Verification items for the finished model (mm, model axes). A direction names the side the tool comes from. Give positions to 0.01 mm unless a question says otherwise; leave off trailing zeros. Loops run counter-clockwise (first coordinate to the right, second up) from the corner with the lowest first, then second, coordinate; pieces in that order, holes last. Notation, with made-up numbers: M 40,63 L 96,63 A17 ccw 96,87 Z; hole C -27,-27 d10. An arc over 180 degrees is marked long. Answer in a Markdown table with one row per item.
```python
from build123d import *

# Parameters (mm, degrees)
SKETCH1_W           = 28.575
SKETCH1_H           = 28.575
BOSS_EXTRUDE1_DEPTH = 1.5875
SKETCH2_R           = 7.9375
BOSS_EXTRUDE2_DEPTH = 3.175
SKETCH3_R           = 11.1125
BOSS_EXTRUDE3_DEPTH = 12.7
FILLET1_R           = 1.27
DOME1_FACE_RADIUS   = 9.8425
DOME1_HEIGHT        = 6.35
FILLET2_R           = 1.27


with BuildPart() as part:
    # Sketch1 → Boss-Extrude1 (new body)
    with BuildSketch(Plane(origin=(0, 0, 0), x_dir=(1, 0, 0), z_dir=(0, 1, 0))):
        Rectangle(SKETCH1_W, SKETCH1_H)
    extrude(amount=BOSS_EXTRUDE1_DEPTH)

    # Sketch2 → Boss-Extrude2 (add)
    with BuildSketch(Plane(origin=(0, 1.5875, 0), x_dir=(1, 0, 0), z_dir=(0, 1, 0))):
        Circle(SKETCH2_R)
    extrude(amount=BOSS_EXTRUDE2_DEPTH)

    # Sketch3 → Boss-Extrude3 (add)
    with BuildSketch(Plane.XZ):
        Circle(SKETCH3_R)
    extrude(amount=BOSS_EXTRUDE3_DEPTH)

    # Fillet1
    fillet1_edges = [part.edges().sort_by_distance(p)[0] for p in [
        (-7.9375, 4.7625, 0),
        (-11.1125, -12.7, 0),
    ]]
    fillet(fillet1_edges, radius=FILLET1_R)

    # Dome1: a dome of height H over a round flat face of radius A is a cap of a sphere of radius (A * A + H * H) / (2 * H)
    dome1_r = (DOME1_FACE_RADIUS * DOME1_FACE_RADIUS + DOME1_HEIGHT * DOME1_HEIGHT) / (2 * DOME1_HEIGHT)
    dome1_base = Plane((0, -12.7, 0), z_dir=(0, -1, 0))
    with Locations(dome1_base.offset(DOME1_HEIGHT - dome1_r)):
        dome1_ball = Sphere(dome1_r, mode=Mode.PRIVATE)
    add(split(dome1_ball, bisect_by=dome1_base, keep=Keep.TOP, mode=Mode.PRIVATE))

    # Fillet2
    fillet2_edges = [part.edges().sort_by_distance(p)[0] for p in [
        (14.2875, 0.79375, 14.2875),
        (-14.2875, 0.79375, 14.2875),
        (-14.2875, 0.79375, -14.2875),
        (14.2875, 0.79375, -14.2875),
    ]]
    fillet(fillet2_edges, radius=FILLET2_R)


solid = part.part
```
Item 1: Sectioned sample at C-C (y = -0.75). Record the cut outline in (x, z) (1 decimal).
Reported:
| item | result |
|---|---|
| outline | C 0,0 d22.2 |
Item 2: Sectioned sample at A-A (z = 0). Record the cut outline in (x, y).
Reported:
| item | result |
|---|---|
| outline | M -14.29,0 L -11.11,0 L -11.11,-11.43 A1.27 ccw -9.84,-12.7 A10.8 ccw 9.84,-12.7 A1.27 ccw 11.11,-11.43 L 11.11,0 L 14.29,0 L 14.29,1.59 L 7.94,1.59 L 7.94,3.49 A1.27 ccw 6.67,4.76 L -6.67,4.76 A1.27 ccw -7.94,3.49 L -7.94,1.59 L -14.29,1.59 Z |
Item 3: Go/stop test with flat-tipped pins: pin 1 (3 mm diameter, centred on y = -7.5, z = 6.5, fed in from -X); pin 2 (6 mm diameter, centred on x = 9, y = -13.5, fed in from -Z); pin 3 (14.5 mm diameter, centred on x = 6.5, z = -3.5, fed in from -Y). Record where each tip stops, or that it passes through.
Reported:
| item | result |
|---|---|
| pin 1 | stops at x = -9.92 |
| pin 2 | stops at z = -8.93 |
| pin 3 | stops at y = -19.05 |
Item 4: Sectioned sample at B-B (x = 0). Record the cut outline in (y, z).
Reported:
| item | result |
|---|---|
| outline | M -12.7,-9.84 A1.27 ccw -11.43,-11.11 L 0,-11.11 L 0,-14.29 L 1.59,-14.29 L 1.59,-7.94 L 3.49,-7.94 A1.27 ccw 4.76,-6.67 L 4.76,6.67 A1.27 ccw 3.49,7.94 L 1.59,7.94 L 1.59,14.29 L 0,14.29 L 0,11.11 L -11.43,11.11 A1.27 ccw -12.7,9.84 A10.8 ccw Z |
Item 5: Scan lines: L1, parallel to Y at x = 13, z = -4.5; L2, parallel to Y at x = -7.75, z = -6.25; L3, parallel to X at y = -17, z = 0. Record each from-to range of solid material in increasing order. Write a range as [from, to].
Reported:
| item | result |
|---|---|
| L1 | y = [0, 1.59] |
| L2 | y = [-12.69, 1.59] |
| L3 | x = [-6.33, 6.33] |
Item 6: Sectioned sample at D-D (y = -13.5). Record the cut outline in (x, z).
Reported:
| item | result |
|---|---|
| outline | C 0,0 d18.88 |
Item 7: Tool access check on faces 1 (the cylindrical face through (-1.72, 2.53, 7.75)), 2 (the flat face through (0, 1, -14.288)), 3 (the cylindrical face through (10.6, -5.63, 3.34)). Record the directions out of +Z, -Z, +X, -X, +Y, -Y that give a thin tool (end or side, any length) a straight path to the whole face; none if there is none.
Reported:
| item | result |
|---|---|
| face 1 | +Y |
| face 2 | -Z, +X, -X, +Y, -Y |
| face 3 | -Y |
